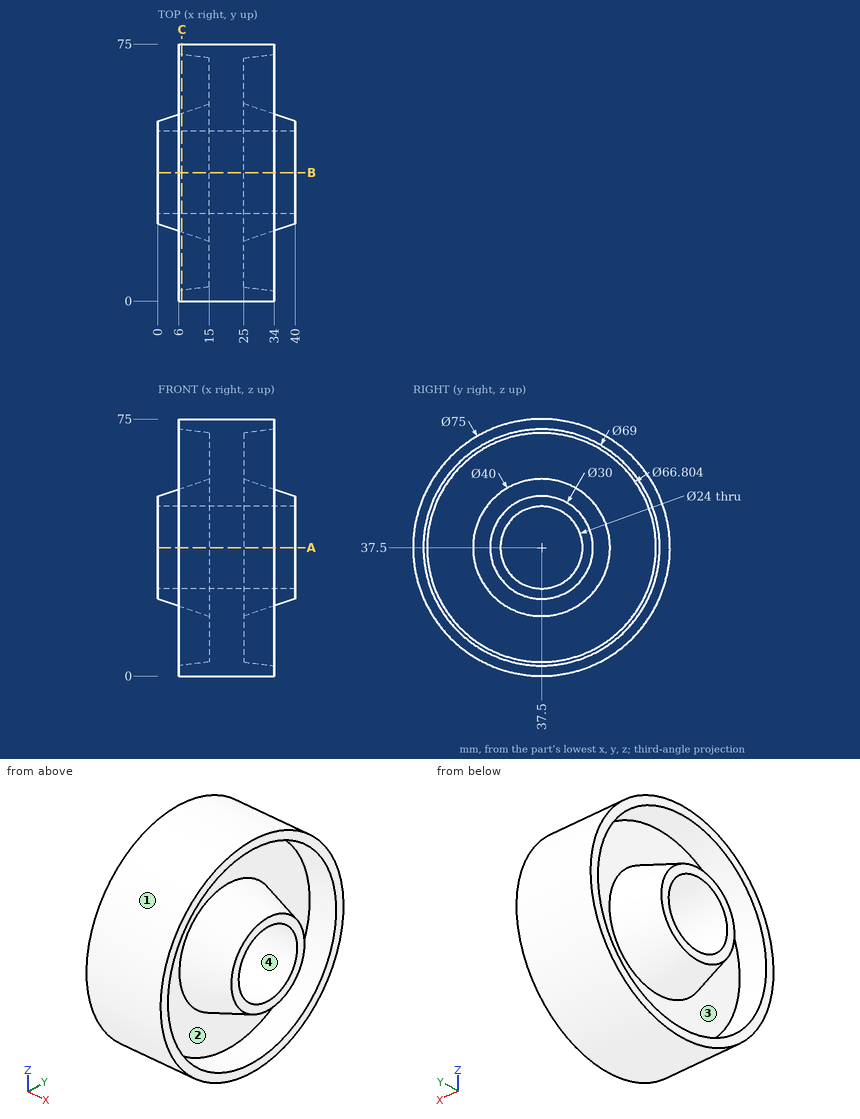
Here's the drawing with two shaded views (mm, measured from the low corner). I have some questions. A direction names the side the tool comes from. Coordinates: 2 decimals unless noted, no trailing zeros. Order: outer loops, then holes, each group sorted by start corner. A loop starts at its lowest first (then second) coordinate and runs counter-clockwise, first axis right, second up.
Q1. Thinking about a two-plate mould opening in Z: for the marked faces 1 and 2, which applies, released by +Z, released by -Z, zero draft, split by the parting line, or undercut?
Q2. Which directions (+Z, -Z, +X, -X, +Y, -Y) give clear straight access to the entire face, cutting with the end or side of a thin tool? Please do the marked faces 3 and 4.
Q3. Please list where these lines run through material, in increasing order: L1, parallel to Y at x = 19, z = 37.5; L2, parallel to Z at x = 22, y = 38; L3, parallel to Y at x = 29, z = 37.5.
Q4. Suppose I cut it at C-C on x = 7. Please give me the cut outline in (y, z), and give its area (3 significant figures).
Q5. Will these pins go through, and if not, where does the flat tip stop? pin 1 (1 mm diameter, centred on x = 29, y = 41.5, fed in from -Z); pin 2 (8 mm diameter, centred on x = 26, y = 62.5, fed in from +Z); pin 3 (2 mm diameter, centred on x = 8, z = 17.5, fed in from +Y).
Q6. Suppose I cut it at A-A on z = 37.5. Please give me the cut outline in (x, y).
Answer:
1. face 1: split by the parting line
1. face 2: undercut
2. face 3: -X
2. face 4: +X, -X
3. L1: y = 0 to 25.5, 49.5 to 75
3. L2: z = 0 to 25.51, 49.49 to 75
3. L3: y = 0 to 3.61, 18.83 to 25.5, 49.5 to 56.17, 71.39 to 75
4. outline: circle Ø75 at (37.5, 37.5); circle Ø34.67 at (37.5, 37.5); hole circle Ø68.76 at (37.5, 37.5); hole circle Ø24 at (37.5, 37.5)
4. area: 1,200 mm2
5. pin 1: stops at z = 0.16
5. pin 2: stops at z = 68.57
5. pin 3: stops at y = 69.83
6. outline: (0, 22.5) - (15, 17.5) - (15, 4.1) - (6, 3) - (6, 0) - (34, 0) - (34, 3) - (25, 4.1) - (25, 17.5) - (40, 22.5) - (40, 25.5) - (0, 25.5) - close; (0, 49.5) - (40, 49.5) - (40, 52.5) - (25, 57.5) - (25, 70.9) - (34, 72) - (34, 75) - (6, 75) - (6, 72) - (15, 70.9) - (15, 57.5) - (0, 52.5) - close
